Can you work these out from the model? Positions are in its coordinate system, mm. Face numbers are marked on the shaded views. A direction names the side the tool comes from. Give positions to 0.01 mm unless a question says otherwise; leave off trailing zeros. Loops run counter-clockwise (first coordinate to the right, second up) from the corner with the lowest first, then second, coordinate; pieces in that order, holes last. Notation, with made-up numbers: M 80,-33 L 131,-33 A20 cw 131,-26 Z; hole C -34,44.5 d1. An arc over 180 degrees is marked long. Put each result on its own line as item: value. Start each with the question number.
1) For the marked faces 1, 2 and 3, which set-ups out of +Z, -Z, +X, -X, +Y, -Y let a thin tool reach every point of the face, with its end or its side?
2) Imagine slicing it at B-B (z = -6.5). Write out the boundary of the cut face in (x, y), then the cut area to 3 significant figures.
3) Imagine slicing it at A-A (x = 1.55). Write out the boundary of the cut face in (y, z), then the cut area to 3 significant figures.
4) Please list where this line runs through material, in increasing order: line 1 along Y through (x, z) = (0.15, 5.5). Write a range as from..to.
5) For P1, Ø0.8, axis at x = 1, z = -6.5, coming from the +Y side; P2, Ø1.5, axis at x = 1.5, y = -18, coming from the -Z side; P3, Ø1.2, axis at x = 1.5, z = -6.5, coming from the -Y side, each with a flat end and sliding along its axis, tell me the tip position at first contact or that it passes through.
Autodesk Inventor part; units mm, degrees
ref_plane "YZ Plane" through (0, 0, 0) normal (1, 0, 0) x (0, 1, 0)
ref_plane "XZ Plane" through (0, 0, 0) normal (0, 1, 0) x (-1, 0, 0)
ref_plane "XY Plane" through (0, 0, 0) normal (0, 0, 1) x (1, 0, 0)
sketch "Sketch1" plane through (0, 0, 0) normal (1, 0, 0) x (0, 1, 0)
  line L0 (-16, -7.5) -> (16, -7.5)
  line L1 (16, -7.5) -> (16, 7.5)
  line L2 (16, 7.5) -> (-16, 7.5)
  line L3 (-16, 7.5) -> (-16, -7.5)
  line L4 (-16, -7.5) -> (16, 7.5) construction
  line L5 (16, -7.5) -> (-16, 7.5) construction
  point P0 (0, 0)
  dimension "d0" = 32
  dimension "d1" = 15
extrude "Extrusion1" add sketch "Sketch1" along normal blind 3
sketch "Sketch2" plane through (3, 0, 0) normal (1, 0, 0) x (0, 0, -1)
  line L0 (7.5, 16) -> (-7.5, 16)
  line L1 (-5, 16) -> (5, 16)
  line L2 (5, 16) -> (5, 19)
  line L3 (5, 19) -> (-5, 19)
  line L4 (-5, 19) -> (-5, 16)
  line L5 (-5, -16) -> (5, -16)
  line L6 (5, -16) -> (5, -19)
  line L7 (5, -19) -> (-5, -19)
  line L8 (-5, -19) -> (-5, -16)
  line L9 (-7.5, -16) -> (7.5, -16)
  point P0 (0, 0)
  point P1 (0, 19)
  dimension "d4" = 10
  dimension "d5" = 3
  dimension "d6" = 10
  dimension "d7" = 3
extrude "Extrusion2" add sketch "Sketch2" against normal blind 3
properties part number "Mid rib support"
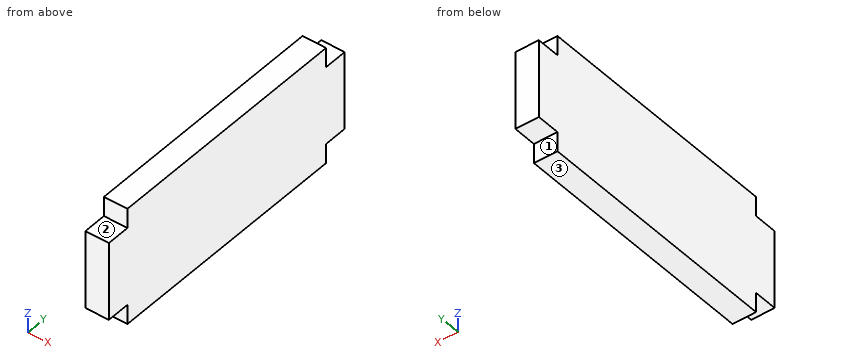
Recorded:
1. face 1: -Z, +X, -X, +Y
1. face 2: +Z, +X, -X, -Y
1. face 3: -Z, +X, -X, +Y, -Y
2. outline: M 0,-16 L 3,-16 L 3,16 L 0,16 Z
2. area: 96.0 mm²
3. outline: M -19,-5 L -16,-5 L -16,-7.5 L 16,-7.5 L 16,-5 L 19,-5 L 19,5 L 16,5 L 16,7.5 L -16,7.5 L -16,5 L -19,5 Z
3. area: 540 mm²
4. line 1: -16..16
5. P1: y = 16
5. P2: z = -5
5. P3: y = -16
